Build history of the part. All positions in model axes, mm. Face numbers are marked on the shaded views. A direction names the side the tool comes from. Round coordinates to 2 decimals unless told otherwise and drop trailing zeros. Order: outer loops, then holes, each group sorted by start corner. A loop starts at its lowest first (then second) coordinate and runs counter-clockwise, first axis right, second up. Notation, with made-up numbers: (-21, 52.5) -> (14, 52.5) arc R30 cw to (14, 78.5) -> close; hole circle Ø4 at (55.5, 72.25). An arc over 180 degrees is marked (long way). Write item = value, one per line.
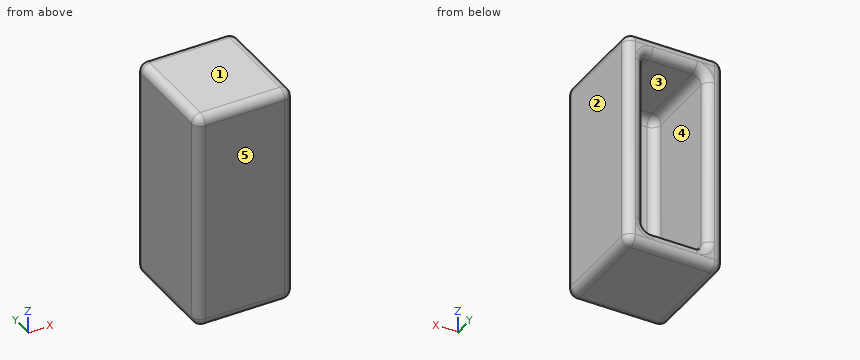
Autodesk Inventor part; units mm, degrees
ref_plane "YZ Plane" through (0, 0, 0) normal (1, 0, 0) x (0, 1, 0)
ref_plane "XZ Plane" through (0, 0, 0) normal (0, 1, 0) x (-1, 0, 0)
ref_plane "XY Plane" through (0, 0, 0) normal (0, 0, 1) x (1, 0, 0)
sketch "Sketch1" plane through (0, 0, 0) normal (0, 1, 0) x (-1, 0, 0)
  line L0 (0, 0) -> (-7, 0)
  line L1 (-7, 0) -> (-7, -21)
  line L2 (-7, -21) -> (0, -21)
  line L3 (0, -21) -> (0, 0)
  line L4 (0, 0) -> (2, 0)
  line L5 (2, 0) -> (2, 2)
  line L6 (2, 2) -> (0, 2)
  line L7 (0, 2) -> (0, 0)
  line L8 (-7, -21) -> (-9, -21)
  line L9 (-9, -21) -> (-9, -23)
  line L10 (-9, -23) -> (-7, -23)
  line L11 (-7, -23) -> (-7, -21)
  line L12 (-9, -23) -> (2, -23)
  line L13 (2, -23) -> (2, 2)
  line L14 (2, 2) -> (-9, 2)
  line L15 (-9, 2) -> (-9, -23)
  dimension "d0" = 7
  dimension "d1" = 21
  dimension "d2" = 2
  dimension "d3" = 2
  dimension "d4" = 2
  dimension "d5" = 2
extrude "Extrusion1" add sketch "Sketch1" along normal blind 2
sketch "Sketch2" plane through (0, 2, 0) normal (0, 1, 0) x (1, 0, 0)
  line L0 (-2, -2) -> (9, -2)
  line L1 (-2, -2) -> (0, -2)
  line L2 (0, -2) -> (0, 0)
  line L3 (0, 0) -> (-2, 0)
  line L4 (-2, 0) -> (-2, -2)
  line L5 (9, -2) -> (9, 23)
  line L6 (9, 23) -> (7, 23)
  line L7 (7, 23) -> (7, 21)
  line L8 (7, 21) -> (9, 21)
  line L9 (9, 21) -> (9, 23)
  line L10 (0, 0) -> (7, 0)
  line L11 (7, 0) -> (7, 21)
  line L12 (7, 21) -> (0, 21)
  line L13 (0, 21) -> (0, 0)
  line L14 (-2, 23) -> (-2, -2)
  line L15 (-2, -2) -> (9, -2)
  line L16 (9, -2) -> (9, 23)
  line L17 (9, 23) -> (-2, 23)
  line L18 (-2, 23) -> (-2, -2)
  dimension "d8" = 2
  dimension "d9" = 2
  dimension "d10" = 2
  dimension "d11" = 2
extrude "Extrusion2" add sketch "Sketch2" along normal blind 10 contours L4 L3 L2 L0 | L2 L10 L11 L8 L5 L0 | L14 L17 L7 L12 L13 L3 | L8 L7 L6 L5
fillet "Fillet1" radius 1 8 edges at (0, 7, -21) (0, 7, 0) (7, 7, 0) (7, 7, -21) (9, 6, 2) (-2, 6, 2) (-2, 6, -23) (9, 6, -23)
fillet "Fillet2" radius 1 32 edges at (0.2929, 2, -0.2929) (3.5, 2, 0) (6.7071, 2, -0.2929) (7, 2, -10.5) (6.7071, 2, -20.7071) (3.5, 2, -21) (0.2929, 2, -20.7071) (0, 2, -10.5) (6.7071, 12, -20.7071) (7, 12, -10.5) (6.7071, 12, -0.2929) (3.5, 12, 0) (0.2929, 12, -0.2929) (0, 12, -10.5) (0.2929, 12, -20.7071) (3.5, 12, -21) (-1.7071, 12, -22.7071) (-2, 12, -10.5) (-1.7071, 12, 1.7071) (3.5, 12, 2) (8.7071, 12, 1.7071) (9, 12, -10.5) (8.7071, 12, -22.7071) (3.5, 12, -23) (8.7071, 0, -22.7071) (3.5, 0, -23) (-1.7071, 0, -22.7071) (-2, 0, -10.5) (-1.7071, 0, 1.7071) (3.5, 0, 2) (8.7071, 0, 1.7071) (9, 0, -10.5)
properties part number "MechanicalPencilLeadCap"
Q1. Probe probe 1 along X at (y, z) = (10.5, -19.75); probe 2 along Z at (x, y) = (4, 5.5); probe 3 along Y at (x, z) = (5.25, -19). List the from-to ranges inside material, lowest first.
Check values:
probe_1 = -2 to 0, 7 to 9
probe_2 = -23 to -21, 0 to 2
probe_3 = 0 to 2
Q2. Flat gauge pin, fed straight in: pin 1 (1.5 mm diameter, centred on x = 3, z = -7, fed in from +Y). Where does the tip first touch, or does it go through?
Check values:
pin_1 = 2
Q3. Which spindle directions (+Z, -Z, +X, -X, +Y, -Y) get a long thin tool onto all of the face, cutting with end or side? Do the marked faces 4 and 5. Say none if no direction does.
Check values:
face_4 = +Y
face_5 = +Z, -Z, +X, -X, -Y
Q4. Mould opens along X. For the marked faces 1, 2 and 3 say: released by +X, released by -X, zero draft, split by the parting line, or undercut.
Check values:
face_1 = zero draft
face_2 = released by +X
face_3 = undercut
Q5. Cut at A-A, the plane y = 8.75. List the corners of the cut face in (x, z).
Check values:
outline = (-2, -22) arc R1 ccw to (-1, -23) -> (8, -23) arc R1 ccw to (9, -22) -> (9, 1) arc R1 ccw to (8, 2) -> (-1, 2) arc R1 ccw to (-2, 1) -> close; hole (0, -20) arc R1 ccw to (1, -21) -> (6, -21) arc R1 ccw to (7, -20) -> (7, -1) arc R1 ccw to (6, 0) -> (1, 0) arc R1 ccw to (0, -1) -> close
